For this review, take the finished solid that the model builds, in its own axes (mm). Give positions to 0.01 mm unless a question says otherwise; leave off trailing zeros. Write each loop counter-clockwise with the first axis right and the second up, starting at its lowest first coordinate (ties: lowest second). Pieces come first, ordered by that corner, then holes. Notation, with made-up numbers: M 3.5,-37.5 L 48.5,-37.5 A24 ccw 48.5,-8.5 Z; hole C 9.25,34 d2. An arc over 180 degrees is marked long. Use one line per item in the form item = value. Start each with the question number.
Q1. Consider section A-A on y = 0. Write out the cut boundary in (x, z).
Q2. For probe 1 along Y at (x, z) = (2.7, 0); probe 2 along Z at (x, y) = (1.5, 7.5); probe 3 along Z at (x, y) = (2.5, 45), list the stretches that pass through material, from the lowest coordinate up. Write a range as [from, to].
Q3. Clearance check with flat-ended pins moving along their axes: pin 1 Ø1.5 at (x, y) = (2.5, 1) entering from +Z; pin 2 Ø3 at (x, y) = (1.5, 39) entering from -Z; pin 3 Ø1.5 at (x, y) = (3, -24.5) entering from -Z; pin 4 Ø3 at (y, z) = (45, 0) entering from +X. State where each tip first meets the part, or that it passes through.
Q4. Consider section C-C on x = 1.6. Write out the cut boundary in (y, z), and give its area (3 significant figures).
Q5. Consider section D-D on z = -23. Write out the cut boundary in (x, y), and give its area (3 significant figures).
Q6. Consider section B-B on z = 0. Write out the cut boundary in (x, y), and give its area (3 significant figures).
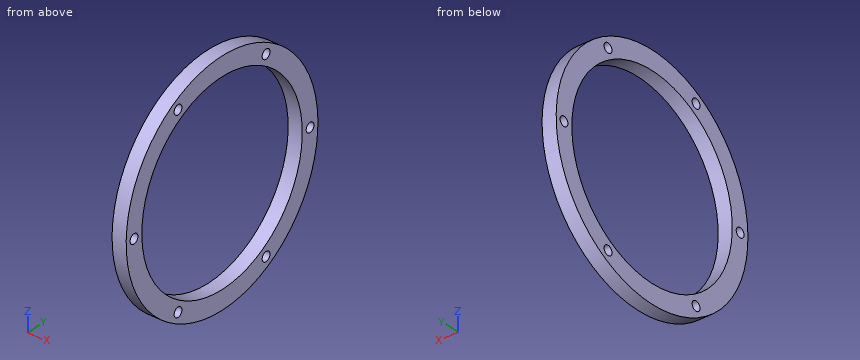
```python
from build123d import *

# Parameters (mm, degrees)
SKETCH1_R           = 49
SKETCH1_R_2         = 41
BOSS_EXTRUDE1_DEPTH = 6
CIRPATTERN1_COUNT   = 6


with BuildPart() as part:
    # Sketch1 → Boss-Extrude1 (new body)
    with BuildSketch(Plane(origin=(0, 0, 0), x_dir=(0, 0, -1), z_dir=(1, 0, 0))):
        Circle(SKETCH1_R)
        Circle(SKETCH1_R_2, mode=Mode.SUBTRACT)
    extrude(amount=BOSS_EXTRUDE1_DEPTH)

    # Sketch3 → Ø4.0mm Dowel Hole1 (revolve, cut)
    with BuildSketch(Plane(origin=(6, 45, 0), x_dir=(0, 0, -1), z_dir=(0, 1, 0))):
        Polygon((0, 0), (0, 51.201721238), (2, 50), (2, 0), align=None)
    f_4_0mm_dowel_hole1 = revolve(axis=Axis((12.35, 45, 0), (-1, 0, 0)), mode=Mode.SUBTRACT)

    # CirPattern1: Ø4.0mm Dowel Hole1 ×6 about axis
    cirpattern1_axis = Axis((0, 0, 0), (1, 0, 0))
    for i in range(1, CIRPATTERN1_COUNT):
        add(f_4_0mm_dowel_hole1.rotate(cirpattern1_axis, i * 360 / CIRPATTERN1_COUNT), mode=Mode.SUBTRACT)


solid = part.part
```
Working result:
q1.outline = M 0,-49 L 6,-49 L 6,-41 L 0,-41 Z; M 0,41 L 6,41 L 6,49 L 0,49 Z
q2.probe_1 = [-49, -47], [-43, -41], [41, 43], [47, 49]
q2.probe_2 = [-48.42, -40.31], [40.31, 48.42]
q2.probe_3 = [-19.39, -2], [2, 19.39]
q3.pin_1 = 49
q3.pin_2 = -31.54
q3.pin_3 = -42.86
q3.pin_4 = through
q4.outline = C 0,0 d98; hole C -45,0 d4; hole C 0,0 d82; hole C -22.5,-38.97 d4; hole C -22.5,38.97 d4; hole C 22.5,-38.97 d4; hole C 22.5,38.97 d4; hole C 45,0 d4
q4.area = 2,190 mm²
q5.outline = M 0,-43.27 L 6,-43.27 L 6,-33.94 L 0,-33.94 Z; M 0,33.94 L 6,33.94 L 6,43.27 L 0,43.27 Z
q5.area = 112 mm²
q6.outline = M 0,-49 L 6,-49 L 6,-47 L 0,-47 Z; M 0,-43 L 6,-43 L 6,-41 L 0,-41 Z; M 0,41 L 6,41 L 6,43 L 0,43 Z; M 0,47 L 6,47 L 6,49 L 0,49 Z
q6.area = 48.0 mm²
